from build123d import *

# Parameters (mm, degrees)
F0_W     = 30
F0_H     = 80
F1_DEPTH = 6
F2_R     = 5
F3_R     = 5
F4_R     = 5
F5_R     = 5
F6_R     = 2.5
F7_R     = 2.5
F9_D     = 20
F13_D    = 20
F14_D    = 20


with BuildPart() as f1:
    # F0 (on Front) → F1 (new body)
    with BuildSketch(Plane.XZ):
        with Locations((15, 40)):
            Rectangle(F0_W, F0_H)
    extrude(amount=F1_DEPTH)

    # F2
    f2_edges = [f1.edges().sort_by_distance(p)[0] for p in [
        (30, -3, 80),
    ]]
    fillet(f2_edges, radius=F2_R)

    # F3
    f3_edges = [f1.edges().sort_by_distance(p)[0] for p in [
        (0, -3, 80),
    ]]
    fillet(f3_edges, radius=F3_R)

    # F4
    f4_edges = [f1.edges().sort_by_distance(p)[0] for p in [
        (0, -3, 0),
    ]]
    fillet(f4_edges, radius=F4_R)

    # F5
    f5_edges = [f1.edges().sort_by_distance(p)[0] for p in [
        (30, -3, 0),
    ]]
    fillet(f5_edges, radius=F5_R)

    # F6
    f6_edges = [f1.edges().sort_by_distance(p)[0] for p in [
        (28.535534, -6, 78.535534),
    ]]
    fillet(f6_edges, radius=F6_R)

    # F7
    f7_edges = [f1.edges().sort_by_distance(p)[0] for p in [
        (28.535534, 0, 78.535534),
    ]]
    fillet(f7_edges, radius=F7_R)

    # F9 (through all)
    with Locations(Plane.XZ.offset(6)):
        with Locations((15, 40)):
            Hole(F9_D / 2)

    # F13 (through all)
    with Locations(Plane.XZ.offset(6)):
        with Locations((15.093754977, 65)):
            Hole(F13_D / 2)

    # F14 (through all)
    with Locations(Plane.XZ.offset(6)):
        with Locations((15.093754977, 14.9996483952)):
            Hole(F14_D / 2)


solid = f1.part
Source: CAD feature listing. Evaluate the final solid. Frame: model axes, mm. Give positions to 0.01 mm unless a question says otherwise; leave off trailing zeros. Write each loop counter-clockwise with the first axis right and the second up, starting at its lowest first coordinate (ties: lowest second). Pieces come first, ordered by that corner, then holes. Notation, with made-up numbers: (56, 54.25) -> (113, 54.25) arc R22 ccw to (113, 72.25) -> close; hole circle Ø11 at (-19.75, -14). An arc over 180 degrees is marked (long way). Write item = value, one per line.
Q1. Cut plane B-B on x = 15. Return loops of the section in (y, z).
Here are the results:
outline = (-6, 2.5) arc R2.5 ccw to (-3.5, 0) -> (-2.5, 0) arc R2.5 ccw to (0, 2.5) -> (0, 5) -> (-6, 5) -> close; (-6, 25) -> (0, 25) -> (0, 30) -> (-6, 30) -> close; (-6, 50) -> (0, 50) -> (0, 55) -> (-6, 55) -> close; (-6, 75) -> (0, 75) -> (0, 77.5) arc R2.5 ccw to (-2.5, 80) -> (-3.5, 80) arc R2.5 ccw to (-6, 77.5) -> close
Q2. Mould query, pull axis X, two halves, no side actions, for faces 1 (the face through (5.556, -2.958, 18.003)), 2 (the face through (29.248, -0.713, 40.49)), 3 (the face through (14.86, -0.713, 79.248)), 4 (the face through (10.386, -2.958, 31.128)). Classes: +X half, -X half, draft (parallel to the pull), parting line (faces both ways), or undercut.
Here are the results:
face_1 = undercut
face_2 = +X half
face_3 = draft
face_4 = undercut
Q3. Cut plane A-A on z = 65. Return loops of the section in (x, y).
Here are the results:
outline = (0, -3.5) arc R2.5 ccw to (2.5, -6) -> (5.09, -6) -> (5.09, 0) -> (2.5, 0) arc R2.5 ccw to (0, -2.5) -> close; (25.09, -6) -> (27.5, -6) arc R2.5 ccw to (30, -3.5) -> (30, -2.5) arc R2.5 ccw to (27.5, 0) -> (25.09, 0) -> close
Q4. First-contact query: pin 1 (12 mm diameter, centred on x = 15.09, z = 65, fed in from -Y); pin 2 (1.5 mm diameter, centred on y = -4.5, z = 62, fed in from +X). Flat tips, straight axial feed; report the tip coordinate or a pass-through.
Here are the results:
pin_1 = through
pin_2 = 29.99
Q5. Line query: line 1 (Z direction, x = 14.5, y = -3.8); line 2 (Z direction, x = 20.5, y = -2.3); line 3 (X direction, y = -5.15, z = 58.5). Output: solid intervals per line, ascending. Write a range as from..to.
Here are the results:
line_1 = 0.02..5.02, 24.98..30.01, 49.99..55.02, 74.98..79.98
line_2 = 0.01..6.59, 23.41..31.65, 48.35..56.59, 73.41..79.99
line_3 = 0.62..7.49, 22.69..29.38
Q6. Cut plane D-D on x = 21.75. Return loops of the section in (y, z), then the cut area to 3 significant figures.
Here are the results:
outline = (-6, 2.5) arc R2.5 ccw to (-3.5, 0) -> (-2.5, 0) arc R2.5 ccw to (0, 2.5) -> (0, 7.54) -> (-6, 7.54) -> close; (-6, 22.46) -> (0, 22.46) -> (0, 32.62) -> (-6, 32.62) -> close; (-6, 47.38) -> (0, 47.38) -> (0, 57.54) -> (-6, 57.54) -> close; (-6, 72.46) -> (0, 72.46) -> (0, 77.5) arc R2.5 ccw to (-2.5, 80) -> (-3.5, 80) arc R2.5 ccw to (-6, 77.5) -> close
area = 207 mm²
Q7. Cut plane C-C on z = 10.5. Return loops of the section in (x, y), then the cut area to 3 significant figures.
Here are the results:
outline = (0, -3.5) arc R2.5 ccw to (2.5, -6) -> (6.16, -6) -> (6.16, 0) -> (2.5, 0) arc R2.5 ccw to (0, -2.5) -> close; (24.02, -6) -> (27.5, -6) arc R2.5 ccw to (30, -3.5) -> (30, -2.5) arc R2.5 ccw to (27.5, 0) -> (24.02, 0) -> close
area = 67.5 mm²
